```python
from build123d import *

# Parameters (mm, degrees)
F0_W      = 28
F0_H      = 28
F1_DEPTH  = 31.5
F2_R      = 11
F3_DEPTH  = 1.5
F4_R      = 2.5
F5_DEPTH  = 18.5
F6_SIZE   = 1.5
F7_SIZE   = 0.3
F8_R      = 1.49999
F10_DEPTH = 31.5


# Not quite as in the source:
# - a fillet or chamfer is up to 0.001 mm smaller than in the source, because OpenCascade refuses the exact size


with BuildPart() as f1:
    # F0 (on Front) → F1 (new body)
    with BuildSketch(Plane.XZ):
        Rectangle(F0_W, F0_H)
    extrude(amount=-F1_DEPTH)

    # F2 (on face) → F3 (join)
    with BuildSketch(Plane(origin=(0, 31.5, 0), x_dir=(-1, 0, 0), z_dir=(0, 1, 0))):
        Circle(F2_R)
    extrude(amount=F3_DEPTH)

    # F4 (on face) → F5 (join)
    with BuildSketch(Plane(origin=(0, 33, 0), x_dir=(-1, 0, 0), z_dir=(0, 1, 0))):
        Circle(F4_R)
    extrude(amount=F5_DEPTH)

    # F6
    f6_edges = [f1.edges().sort_by_distance(p)[0] for p in [
        (14, 15.75, 14),
        (14, 15.75, -14),
        (-14, 15.75, -14),
        (-14, 15.75, 14),
    ]]
    chamfer(f6_edges, length=F6_SIZE)

    # F7
    f7_edges = [f1.edges().sort_by_distance(p)[0] for p in [
        (2.5, 51.5, 0),
    ]]
    chamfer(f7_edges, length=F7_SIZE)

    # F8 (radius 1.5 in the source; OpenCascade refuses exactly that, so slightly less here)
    f8_edges = [f1.edges().sort_by_distance(p)[0] for p in [
        (11, 33, 0),
    ]]
    fillet(f8_edges, radius=F8_R)

    # F9 (on face) → F10 (cut)
    with BuildSketch(Plane(origin=(0, 31.5, 0), x_dir=(-1, 0, 0), z_dir=(0, 1, 0))):
        with BuildLine():
            Line((-11.5, -11.5), (-11.5, -10.2))
            ThreePointArc((-11.5, -10.2), (-12.4192388155, -12.4192388155), (-10.2, -11.5))
            Line((-10.2, -11.5), (-11.5, -11.5))
        make_face()
        with BuildLine():
            ThreePointArc((-10.2, -11.5), (-10.5807611845, -10.5807611845), (-11.5, -10.2))
            Line((-11.5, -10.2), (-11.5, -11.5))
            Line((-11.5, -11.5), (-10.2, -11.5))
        make_face()
        with BuildLine():
            ThreePointArc((12.8, -11.5), (12.4192388155, -10.5807611845), (11.5, -10.2))
            Line((11.5, -10.2), (11.5, -11.5))
            Line((11.5, -11.5), (10.2, -11.5))
            ThreePointArc((10.2, -11.5), (11.5, -12.8), (12.8, -11.5))
        make_face()
        with BuildLine():
            Line((11.5, -11.5), (11.5, -10.2))
            ThreePointArc((11.5, -10.2), (10.5807611845, -10.5807611845), (10.2, -11.5))
            Line((10.2, -11.5), (11.5, -11.5))
        make_face()
        with BuildLine():
            Line((11.5, 11.5), (10.2, 11.5))
            ThreePointArc((10.2, 11.5), (10.5807611845, 10.5807611845), (11.5, 10.2))
            Line((11.5, 10.2), (11.5, 11.5))
        make_face()
        with BuildLine():
            ThreePointArc((12.8, 11.5), (11.5, 12.8), (10.2, 11.5))
            Line((10.2, 11.5), (11.5, 11.5))
            Line((11.5, 11.5), (11.5, 10.2))
            ThreePointArc((11.5, 10.2), (12.4192388155, 10.5807611845), (12.8, 11.5))
        make_face()
        with BuildLine():
            ThreePointArc((-11.5, 10.2), (-10.5807611845, 10.5807611845), (-10.2, 11.5))
            Line((-10.2, 11.5), (-11.5, 11.5))
            Line((-11.5, 11.5), (-11.5, 10.2))
        make_face()
        with BuildLine():
            Line((-11.5, 11.5), (-10.2, 11.5))
            ThreePointArc((-10.2, 11.5), (-12.4192388155, 12.4192388155), (-11.5, 10.2))
            Line((-11.5, 10.2), (-11.5, 11.5))
        make_face()
    extrude(amount=-F10_DEPTH, mode=Mode.SUBTRACT)


solid = f1.part
```
Input: part model. Units: mm. Frame: model coordinates. A direction names the side the tool comes from. Give positions to 0.01 mm unless a question says otherwise; leave off trailing zeros. Write each loop counter-clockwise with the first axis right and the second up, starting at its lowest first coordinate (ties: lowest second). Pieces come first, ordered by that corner, then holes. Notation, with made-up numbers: (48.5, -9.75) - (62.5, -9.75) arc R31 ccw to (62.5, 26.25) - close; hole circle Ø1 at (-4, 36.25). An arc over 180 degrees is marked (long way). Write item = value, one per line. Start each with the question number.
1) Cut plane C-C (y = 43.5). Return loops of the section in (x, z).
2) Reachability of faces 1 (the face through (0, 51.5, 0)), 2 (the face through (-2, 33, -2)) from +Z, -Z, +X, -X, +Y, -Y: full face, straight path, thin tool, end or side. Return the list, or none.
3) Pin query (flat end, axial travel): pin 1 (3 mm diameter, centred on x = 11.5, z = -11.5, fed in from +Y); pin 2 (1.5 mm diameter, centred on x = 3, y = 33.5, fed in from +Z). Return the tip coordinate at first contact, or that it passes through.
4) Material intervals for L1, parallel to Z at x = 11.5, y = 7; L2, parallel to Z at x = -12.25, y = 17.5, sorted ascending. Write a range as [from, to].
5) Cut plane B-B (y = 12.5). Return loops of the section in (x, z), and give its area (3 significant figures).
Answers follow:
q1.outline = circle Ø5 at (0, 0)
q2.face_1 = +Z, -Z, +X, -X, +Y
q2.face_2 = +Y
q3.pin_1 = 31.5
q3.pin_2 = 9.9
q4.L1 = [-14, -12.8], [-10.2, 10.2], [12.8, 14]
q4.L2 = [-14, -12.56], [-10.44, 10.44], [12.56, 14]
q5.outline = (-14, -12.5) - (-12.5, -14) - (12.5, -14) - (14, -12.5) - (14, 12.5) - (12.5, 14) - (-12.5, 14) - (-14, 12.5) - close; hole circle Ø2.6 at (-11.5, -11.5); hole circle Ø2.6 at (-11.5, 11.5); hole circle Ø2.6 at (11.5, -11.5); hole circle Ø2.6 at (11.5, 11.5)
q5.area = 758 mm^2
